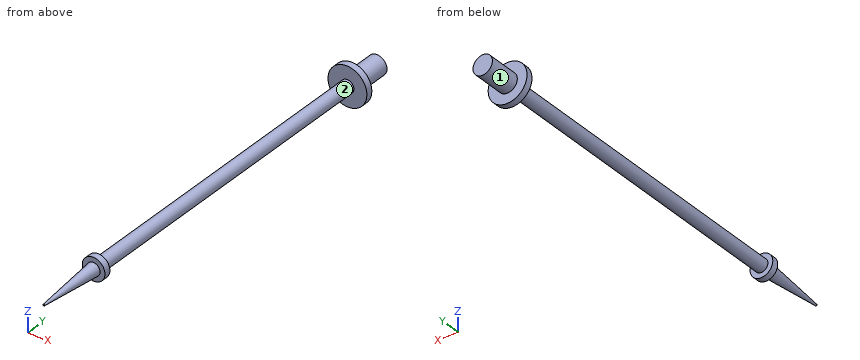
```python
from build123d import *

# Parameters (mm, degrees)
F0_R     = 3
F1_DEPTH = 0.5
F2_R     = 1
F3_DEPTH = 50
F4_R     = 1.5
F5_DEPTH = 5
F6_R     = 1.75
F6_R_2   = 1
F7_DEPTH = 1
F8_R     = 1
F9_DEPTH = 10
F9_TAPER = 5


with BuildPart() as f1:
    # F0 (on Front) → F1 (new body, symmetric)
    with BuildSketch(Plane.XZ):
        Circle(F0_R)
    extrude(amount=F1_DEPTH, both=True)

    # F2 (on face) → F3 (join)
    with BuildSketch(Plane.XZ.offset(0.5)):
        Circle(F2_R)
    extrude(amount=F3_DEPTH)

    # F4 (on face) → F5 (join)
    with BuildSketch(Plane(origin=(0, 0.5, 0), x_dir=(-1, 0, 0), z_dir=(0, 1, 0))):
        Circle(F4_R)
    extrude(amount=F5_DEPTH)

    # F6 (on face) → F7 (join)
    with BuildSketch(Plane.XZ.offset(50.5)):
        Circle(F6_R)
        Circle(F6_R_2, mode=Mode.SUBTRACT)
        Circle(F6_R_2)
    extrude(amount=F7_DEPTH)

    # F8 (on face) → F9 (join)
    with BuildSketch(Plane.XZ.offset(51.5)):
        Circle(F8_R)
    extrude(amount=F9_DEPTH, taper=F9_TAPER)


solid = f1.part
```
Can you work these out from the model? Positions are in its coordinate system, mm. Face numbers are marked on the shaded views. A direction names the side the tool comes from. Coordinates: 2 decimals unless noted, no trailing zeros. Loops run counter-clockwise (first coordinate to the right, second up) from the corner with the lowest first, then second, coordinate; pieces in that order, holes last. Notation, with made-up numbers: M 36.25,-4.5 L 59.25,-4.5 A26 cw 59.25,14.5 Z; hole C 38,72.25 d5. An arc over 180 degrees is marked long. Put each result on its own line as item: value. Start each with the question number.
(1) Imagine slicing it at A-A on y = -13.5. List the corners of the cut face in (x, z) for me.
(2) Imagine slicing it at B-B on x = 2.4. List the corners of the cut face in (y, z) for me, and give its area (3 significant figures).
(3) Will these pins go through, and if not, where does the flat tip stop? pin 1 Ø1 at (x, z) = (-1.5, -0.5) entering from -Y; pin 2 Ø1.5 at (y, z) = (-46.5, 2) entering from -X.
(4) I need wall thicknesses on probe 1 along Y at (x, z) = (0.65, -0.8); probe 2 along Y at (x, z) = (-1.15, -1); probe 3 along X at (y, z) = (-44, 0.1). Which ranges of each line are inside material? Lowest first, please.
(5) Which directions (+Z, -Z, +X, -X, +Y, -Y) give clear straight access to the entire face, cutting with the end or side of a thin tool? Please do the marked faces 1 and 2.
Worked answers:
1. outline: C 0,0 d2
2. outline: M -0.5,-1.8 L 0.5,-1.8 L 0.5,1.8 L -0.5,1.8 Z
2. area: 3.60 mm2
3. pin 1: stops at y = -51.5
3. pin 2: passes through
4. probe 1: y = -51.5 to -50.5, -0.5 to 5.5
4. probe 2: y = -51.5 to -50.5, -0.5 to 0.5
4. probe 3: x = -0.99 to 0.99
5. face 1: +Y
5. face 2: none
